Work out the finished part from the listing and answer in its coordinate system (mm). A direction names the side the tool comes from. Coordinates: 2 decimals unless noted, no trailing zeros. Order: outer loops, then holes, each group sorted by start corner. A loop starts at its lowest first (then second) coordinate and runs counter-clockwise, first axis right, second up. Notation, with made-up numbers: (88, 47) -> (118, 47) arc R27 ccw to (118, 70) -> close; hole circle Ø5 at (31.25, 5). An arc over 180 degrees is marked (long way). Use one line per item in the form item = value.
from build123d import *

# Parameters (mm, degrees)
SZKIC1_R                    = 1
SZKIC1_R_2                  = 1.5
SZKIC1_R_3                  = 1.55
SZKIC1_R_4                  = 2.5
SZKIC1_R_5                  = 5
SZKIC1_R_6                  = 10
SZKIC1_R_7                  = 1.45
SZKIC1_W                    = 25.4
SZKIC1_H                    = 6.4
SZKIC1_H_2                  = 10.4
DODANIE_WYCI_GNI_CIE1_DEPTH = 10


with BuildPart() as part:
    # Szkic1 → Dodanie-wyciągnięcie1 (new body)
    with BuildSketch(Plane(origin=(0, 0, 0), x_dir=(1, 0, 0), z_dir=(0, 1, 0))):
        Polygon((208.426283919, -256.077576053), (233.376283919, -256.077576053), (233.376283919, -281.077576053), (223.376283919, -281.077576053), (223.376283919, -326.077576053), (123.376283919, -326.077576053), (123.376283919, -256.077576053), (138.326283919, -256.077576053), (138.326283919, -259.077576053), (136.951283919, -259.077576053), (136.951283919, -261.077576053), (138.326283919, -261.077576053), (138.326283919, -262.077576053), (141.426283919, -262.077576053), (141.426283919, -261.077576053), (142.801283919, -261.077576053), (142.801283919, -259.077576053), (141.426283919, -259.077576053), (141.426283919, -256.077576053), (151.326283919, -256.077576053), (151.326283919, -263.077576053), (149.951283919, -263.077576053), (149.951283919, -265.077576053), (151.326283919, -265.077576053), (151.326283919, -266.077576053), (154.426283919, -266.077576053), (154.426283919, -265.077576053), (155.801283919, -265.077576053), (155.801283919, -263.077576053), (154.426283919, -263.077576053), (154.426283919, -256.077576053), (160.876283919, -256.077576053), (160.876283919, -250.077576053), (185.876283919, -250.077576053), (185.876283919, -256.077576053), (192.326283919, -256.077576053), (192.326283919, -263.077576053), (190.951283919, -263.077576053), (190.951283919, -265.077576053), (192.326283919, -265.077576053), (192.326283919, -265.577576053), (195.426283919, -265.577576053), (195.426283919, -265.077576053), (196.801283919, -265.077576053), (196.801283919, -263.077576053), (195.426283919, -263.077576053), (195.426283919, -256.077576053), (205.326283919, -256.077576053), (205.326283919, -259.077576053), (203.951283919, -259.077576053), (203.951283919, -261.077576053), (205.326283919, -261.077576053), (205.326283919, -261.577576053), (208.426283919, -261.577576053), (208.426283919, -261.077576053), (209.801283919, -261.077576053), (209.801283919, -259.077576053), (208.426283919, -259.077576053), align=None)
        with Locations(Location((213.376283919, -311.077576053, 0), (0, 0, 270))):
            Circle(SZKIC1_R, mode=Mode.SUBTRACT)
        with Locations(Location((193.376283919, -311.077576053, 0), (0, 0, 270))):
            Circle(SZKIC1_R_2, mode=Mode.SUBTRACT)
        with Locations(Location((183.376283919, -311.077576053, 0), (0, 0, 270))):
            Circle(SZKIC1_R_3, mode=Mode.SUBTRACT)
        with Locations(Location((173.376283919, -311.077576053, 0), (0, 0, 270))):
            Circle(SZKIC1_R_4, mode=Mode.SUBTRACT)
        with Locations(Location((160.376283919, -311.077576053, 0), (0, 0, 270))):
            Circle(SZKIC1_R_5, mode=Mode.SUBTRACT)
        with Locations(Location((140.376283919, -311.077576053, 0), (0, 0, 270))):
            Circle(SZKIC1_R_6, mode=Mode.SUBTRACT)
        with Locations(Location((179.976283919, -279.477576053, 0), (0, 0, 270))):
            Circle(SZKIC1_R_3, mode=Mode.SUBTRACT)
        with Locations(Location((166.976283919, -279.477576053, 0), (0, 0, 270))):
            Circle(SZKIC1_R_3, mode=Mode.SUBTRACT)
        with Locations(Location((179.976283919, -297.877576053, 0), (0, 0, 270))):
            Circle(SZKIC1_R_3, mode=Mode.SUBTRACT)
        with Locations(Location((166.976283919, -297.877576053, 0), (0, 0, 270))):
            Circle(SZKIC1_R_3, mode=Mode.SUBTRACT)
        with Locations(Location((203.376283919, -311.077576053, 0), (0, 0, 270))):
            Circle(SZKIC1_R_7, mode=Mode.SUBTRACT)
        with Locations((200.676283919, -297.877576053)):
            Rectangle(SZKIC1_W, SZKIC1_H, mode=Mode.SUBTRACT)
        with Locations((200.676283919, -279.477576053)):
            Rectangle(SZKIC1_W, SZKIC1_H_2, mode=Mode.SUBTRACT)
        Polygon((161.660555166, -286.935440429), (147.518419543, -272.793304805), (133.376283919, -286.935440429), (147.518419543, -301.077576053), align=None, mode=Mode.SUBTRACT)
    extrude(amount=DODANIE_WYCI_GNI_CIE1_DEPTH)


solid = part.part
(1) Section C-C on x = 157.5 is taken. Write down the section's boundary in (y, z), plus the area to 3 significant figures.
Data:
outline = (0, 256.08) -> (10, 256.08) -> (10, 282.77) -> (0, 282.77) -> close; (0, 291.1) -> (10, 291.1) -> (10, 306.99) -> (0, 306.99) -> close; (0, 315.17) -> (10, 315.17) -> (10, 326.08) -> (0, 326.08) -> close
area = 535 mm²
(2) Straight lines are drawn through the part: line 1 along X through (y, z) = (2, 264); line 2 along Z through (x, y) = (167, 2.5); line 3 along Z through (x, y) = (188.5, 6). For each, find the intervals that lie inside material, in ascending order.
Data:
line_1 = 123.38 to 149.95, 155.8 to 190.95, 196.8 to 233.38
line_2 = 250.08 to 277.93, 281.03 to 296.33, 299.43 to 326.08
line_3 = 256.08 to 274.28, 284.68 to 294.68, 301.08 to 326.08
(3) Which of the six approach directions +Z, -Z, +X, -X, +Y, -Y give full straight-line access (tool end or side, diameter ignored) to faces 1 (the flat face through (228, 5, 281.078)), 2 (the flat face through (140, 5, 262.078)), 3 (the flat face through (154.688, 4.93, 279.963)), 4 (the flat face through (221, 5, 256.078)), 5 (the flat face through (173, 5, 250.078))?
Data:
face_1 = +Z, +X, +Y, -Y
face_2 = -Z, +Y, -Y
face_3 = +Y, -Y
face_4 = -Z, +X, +Y, -Y
face_5 = -Z, +X, -X, +Y, -Y
(4) The mould has two halves that part along Z. Classify faces 6 (the flat face through (195.426, 5, 260)), 7 (the flat face through (146, 5, 256.078)), 8 (the flat face through (200, 5, 284.678)): released by +Z, released by -Z, zero draft, split by the parting line, or undercut.
Data:
face_6 = zero draft
face_7 = released by -Z
face_8 = undercut
(5) Each of these flat-tipped pins is pushed along its axis until it touches: P1, Ø2.5, axis at x = 193.38, z = 311.08, coming from the -Y side; P2, Ø4, axis at x = 193.5, y = 3, coming from the -Z side; P3, Ø0.9, axis at x = 194, y = 3, coming from the -Z side. Where does it stop, or does it pass through?
Data:
P1 = through
P2 = 256.08
P3 = 265.58
(6) Section A-A on x = 211 is taken. Write down the section's boundary in (y, z), plus the area to 3 significant figures.
Data:
outline = (0, 256.08) -> (10, 256.08) -> (10, 274.28) -> (0, 274.28) -> close; (0, 284.68) -> (10, 284.68) -> (10, 294.68) -> (0, 294.68) -> close; (0, 301.08) -> (10, 301.08) -> (10, 326.08) -> (0, 326.08) -> close
area = 532 mm²
(7) Section B-B on z = 291.5 is taken. Write down the section's boundary in (x, y).
Data:
outline = (123.38, 0) -> (137.94, 0) -> (137.94, 10) -> (123.38, 10) -> close; (157.1, 0) -> (223.38, 0) -> (223.38, 10) -> (157.1, 10) -> close
(8) Section D-D on y = 6 is taken. Count the separate pieces of the cut face and the enclosed holes in it, plus the area to 3 significant figures.
Data:
separate_pieces = 1
enclosed_holes = 14
area = 5,990 mm²
